Part model, mm, in its own coordinate system. A direction names the side the tool comes from. Give positions to 0.01 mm unless a question says otherwise; leave off trailing zeros. Order: outer loops, then holes, each group sorted by start corner. A loop starts at its lowest first (then second) coordinate and runs counter-clockwise, first axis right, second up.
1. Drop flat-ended pins along their axis: pin 1 Ø1.6 at (x, z) = (-1.5, 1.5) entering from +Y; pin 2 Ø1 at (y, z) = (-10.5, -5.5) entering from +X; pin 3 Ø5 at (x, y) = (-4, -0.25) entering from -Z; pin 4 Ø6 at (x, y) = (-23.5, 5) entering from -Z. Give the stop position or say it passes through.
2. Slice it at A-A on z = -11. List the corners of the cut face in (x, y).
3. Which spindle directions (+Z, -Z, +X, -X, +Y, -Y) get a long thin tool onto all of the face, cutting with end or side? Do faces 1 (the cylindrical face through (-21.797, -0.127, 3.021)), 2 (the cylindrical face through (-20.4, -14.25, -4.3)), 3 (the flat face through (11, 0.75, -6)), 4 (the cylindrical face through (-1.28, 10.24, 0.15)), 5 (the flat face through (-12, 7, -2.25)). Say none if no direction does.
4. Mould opens along Z. For faces 6 (the flat face through (-21, 3.75, 1)), 7 (the flat face through (-12, 5, -2.25)), 8 (the flat face through (-17.8, -1.5, 1.5)), 9 (the flat face through (10, 6.05, -8)) say: +Z half, -Z half, draft (parallel to the pull), parting line (faces both ways), or undercut.
5. Slice it at B-B on y = -20.25. List the corners of the cut face in (x, z), and give its area (3 significant figures).
6. Probe line 1 (Y direction, x = -19, z = 2.35); line 2 (X direction, y = 1, z = 0.25); line 3 (Z direction, x = -10.5, y = -10). List the from-to ranges inside material, lowest first.
7. Slice it at C-C on y = 11. List the corners of the cut face in (x, z) (3 decimals).
from build123d import *

# Parameters (mm, degrees)
BOSS_EXTRUDE1_DEPTH      = 4.5
SKETCH4_W                = 35.509158229
SKETCH4_H                = 48.512063823
CUT_EXTRUDE2_DEPTH       = 10
SKETCH8_W                = 66
SKETCH8_H                = 9
BOSS_EXTRUDE3_DEPTH      = 5
FILLET7_R                = 10
SKETCH16_R               = 1.5
CUT_EXTRUDE6_DEPTH       = 10
SKETCH17_W               = 15.65
SKETCH17_H               = 52.5
CUT_EXTRUDE7_DEPTH       = 10
SKETCH18_R               = 6
CUT_EXTRUDE8_DEPTH       = 10
SKETCH20_W               = 8
SKETCH20_H               = 28
BOSS_EXTRUDE5_DEPTH      = 18
CUT_EXTRUDE10_DEPTH      = 51.084778127
CUT_EXTRUDE10_DEPTH_BACK = 9
SKETCH23_R               = 8
CUT_EXTRUDE11_DEPTH      = 3
CUT_EXTRUDE12_DEPTH      = 68.0001
CUT_EXTRUDE12_DEPTH_BACK = 8
CUT_EXTRUDE12_START      = -42.7
SKETCH24_W               = 11.249996001
SKETCH24_H               = 2
SKETCH25_R               = 1
CUT_EXTRUDE13_DEPTH      = 12.5
CUT_EXTRUDE15_DEPTH      = 2.25
FILLET8_R                = 4
SKETCH27_W               = 21.7
SKETCH27_H               = 7.5
CUT_EXTRUDE16_DEPTH      = 0.4
CHAMFER1_SIZE            = 0.4
CHAMFER2_SIZE            = 0.4
SKETCH28_R               = 2.8
CUT_EXTRUDE17_DEPTH      = 3
SKETCH29_R               = 2
SKETCH29_W               = 21.7
SKETCH29_H               = 0.8
CUT_EXTRUDE18_DEPTH      = 0.4


# Some blends are built 0.0001 mm under size
with BuildPart() as part:
    # Sketch1 → Boss-Extrude1 (new, symmetric)
    with BuildSketch(Plane.XY):
        Polygon((44.5, -23.75), (-0.5, -23.75), (-44.5, -23.75), (-44.5, 23.75), (44.5, 23.75), align=None)
    extrude(amount=BOSS_EXTRUDE1_DEPTH, both=True)

    # Sketch4 → Cut-Extrude2 (cut)
    with BuildSketch(Plane.XY.offset(4.5)):
        with Locations((39.254579115, -0.506031912)):
            Rectangle(SKETCH4_W, SKETCH4_H)
    extrude(amount=-CUT_EXTRUDE2_DEPTH, mode=Mode.SUBTRACT)

    # Sketch8 → Boss-Extrude3 (add)
    with BuildSketch(Plane(origin=(0, 23.75, 0), x_dir=(1, 0, 0), z_dir=(0, 1, 0))):
        with Locations((-11.5, 0)):
            Rectangle(SKETCH8_W, SKETCH8_H)
    extrude(amount=BOSS_EXTRUDE3_DEPTH)

    # Fillet7
    fillet7_edges = [part.edges().sort_by_distance(p)[0] for p in [
        (-44.5, 28.75, 0),
        (21.5, 28.75, 0),
    ]]
    fillet(fillet7_edges, radius=FILLET7_R)

    # Sketch16 → Cut-Extrude6 (cut)
    with BuildSketch(Plane.XY.offset(4.5)):
        with Locations((-19, -0.25)):
            Circle(SKETCH16_R)
        with Locations((-4, -0.25)):
            Circle(SKETCH16_R)
        with Locations((-19, -20.25)):
            Circle(SKETCH16_R)
        with Locations((-4, -20.25)):
            Circle(SKETCH16_R)
    extrude(amount=-CUT_EXTRUDE6_DEPTH, mode=Mode.SUBTRACT)

    # Sketch17 → Cut-Extrude7 (cut)
    with BuildSketch(Plane(origin=(0, 0, -4.5), x_dir=(-1, 0, 0), z_dir=(0, 0, -1))):
        with Locations((36.675, 2.5)):
            Rectangle(SKETCH17_W, SKETCH17_H)
        with Locations((-13.675, 2.5)):
            Rectangle(SKETCH17_W, SKETCH17_H)
    extrude(amount=-CUT_EXTRUDE7_DEPTH, mode=Mode.SUBTRACT)

    # Sketch18 → Cut-Extrude8 (cut)
    with BuildSketch(Plane.XY.offset(4.5)):
        with Locations((-11.5, 16.25)):
            Circle(SKETCH18_R)
    extrude(amount=-CUT_EXTRUDE8_DEPTH, mode=Mode.SUBTRACT)

    # Sketch20 → Boss-Extrude5 (add)
    with BuildSketch(Plane.XY.offset(4.5)):
        with Locations((-32.85, 14.75)):
            Rectangle(SKETCH20_W, SKETCH20_H)
        with Locations((9.85, 14.75)):
            Rectangle(SKETCH20_W, SKETCH20_H)
    extrude(amount=-BOSS_EXTRUDE5_DEPTH)

    # Sketch22 → Cut-Extrude10 (cut, two sides: drawn at the far end of the back side and taken through both)
    with BuildSketch(Plane.XY.offset(4.5).offset(-CUT_EXTRUDE10_DEPTH_BACK)):
        Polygon((-25, 169.372700937), (-25, 28.75), (-25, 16.25), (2, 16.25), (2, 28.75), (2, 169.372700937), (2, 450.61810281), (-25, 450.61810281), align=None)
    extrude(amount=CUT_EXTRUDE10_DEPTH + CUT_EXTRUDE10_DEPTH_BACK, mode=Mode.SUBTRACT)

    # Sketch23 → Cut-Extrude11 (cut)
    with BuildSketch(Plane(origin=(0, 0, -4.5), x_dir=(-1, 0, 0), z_dir=(0, 0, -1))):
        with Locations((11.5, 16.25)):
            Circle(SKETCH23_R)
    extrude(amount=-CUT_EXTRUDE11_DEPTH, mode=Mode.SUBTRACT)

    # Sketch24 → Cut-Extrude12 (cut, two sides: drawn at the far end of the back side and taken through both)
    with BuildSketch(Plane(origin=(13.85, 0, 0), x_dir=(0, 0, -1), z_dir=(1, 0, 0)).offset(CUT_EXTRUDE12_START - CUT_EXTRUDE12_DEPTH_BACK)):
        with Locations((7.875002, 5.05)):
            Rectangle(SKETCH24_W, SKETCH24_H)
    extrude(amount=CUT_EXTRUDE12_DEPTH + CUT_EXTRUDE12_DEPTH_BACK, mode=Mode.SUBTRACT)

    # Sketch25 → Cut-Extrude13 (cut)
    with BuildSketch(Plane(origin=(0, 16.25, 0), x_dir=(1, 0, 0), z_dir=(0, 1, 0))):
        with Locations(Location((-1.5, -1.125, 0), (0, 0, 180))):
            Circle(SKETCH25_R)
        with Locations(Location((-21.5, -1.125, 0), (0, 0, 180))):
            Circle(SKETCH25_R)
    extrude(amount=-CUT_EXTRUDE13_DEPTH, mode=Mode.SUBTRACT)

    # Sketch26 → Cut-Extrude15 (cut)
    with BuildSketch(Plane(origin=(0, 0, -4.5), x_dir=(-1, 0, 0), z_dir=(0, 0, -1))):
        with BuildLine():
            Line((-5.85, 6.05), (28.85, 6.05))
            Line((28.85, 6.05), (28.85, 28.75))
            Line((28.85, 28.75), (25, 28.75))
            Line((25, 28.75), (25, 16.25))
            Line((25, 16.25), (19.5, 16.25))
            ThreePointArc((19.5, 16.25), (11.5, 8.25), (3.5, 16.25))
            Line((3.5, 16.25), (-2, 16.25))
            Line((-2, 16.25), (-2, 28.75))
            Line((-2, 28.75), (-5.85, 28.75))
            Line((-5.85, 28.75), (-5.85, 6.05))
        make_face()
    extrude(amount=-CUT_EXTRUDE15_DEPTH, mode=Mode.SUBTRACT)

    # Fillet8
    # the kernel refuses this fillet: 4 mm, written as the material it adds along each edge
    with BuildSketch(Plane(origin=(-28.85, 0.75, 4.5), x_dir=(-1, 0, 0), z_dir=(0, 0, -1))) as fillet8_piece_1:
        with BuildLine():
            CenterArc((FILLET8_R, -FILLET8_R), FILLET8_R, 90, 90)
            Line((0, -FILLET8_R), (0, 0))
            Line((0, 0), (FILLET8_R, 0))
        make_face()
    extrude(amount=9)
    with BuildSketch(Plane(origin=(5.85, 0.75, 4.5), x_dir=(1, 0, 0), z_dir=(0, 0, -1))) as fillet8_piece_2:
        with BuildLine():
            CenterArc((FILLET8_R, FILLET8_R), FILLET8_R, 180, 90)
            Line((0, FILLET8_R), (0, 0))
            Line((0, 0), (FILLET8_R, 0))
        make_face()
    extrude(amount=9)
    with BuildSketch(Plane(origin=(2, 16.25, -2.25), x_dir=(-1, 0, 0), z_dir=(0, 0, 1))) as fillet8_piece_3_section:
        with BuildLine():
            CenterArc((FILLET8_R, -FILLET8_R), FILLET8_R, 90, 90)
            Line((0, -FILLET8_R), (0, 0))
            Line((0, 0), (FILLET8_R, 0))
        make_face()
    fillet8_piece_3 = extrude(amount=6.75, mode=Mode.PRIVATE)
    fillet8_piece_3 = fillet8_piece_3 - Plane(origin=(-1.5, 17.15044089, 1.125), x_dir=(-1, 0, 0), z_dir=(0, 1, 0)) * Cylinder(1, 30, mode=Mode.PRIVATE)
    add(fillet8_piece_3)
    with BuildSketch(Plane(origin=(-25, 16.25, -2.25), x_dir=(0, 1, 0), z_dir=(0, 0, 1))) as fillet8_piece_4_section:
        with BuildLine():
            CenterArc((FILLET8_R, -FILLET8_R), FILLET8_R, 90, 90)
            Line((0, -FILLET8_R), (0, 0))
            Line((0, 0), (FILLET8_R, 0))
        make_face()
    fillet8_piece_4 = extrude(amount=6.75, mode=Mode.PRIVATE)
    fillet8_piece_4 = fillet8_piece_4 - Plane(origin=(-21.5, 17.150440868, 1.125), x_dir=(-1, 0, 0), z_dir=(0, 1, 0)) * Cylinder(1, 30, mode=Mode.PRIVATE)
    add(fillet8_piece_4)

    # Sketch27 → Cut-Extrude16 (cut)
    with BuildSketch(Plane(origin=(0, 0, -4.5), x_dir=(-1, 0, 0), z_dir=(0, 0, -1))):
        with Locations((11.5, -20)):
            Rectangle(SKETCH27_W, SKETCH27_H)
        with Locations((11.5, -0.5)):
            Rectangle(SKETCH27_W, SKETCH27_H)
    extrude(amount=-CUT_EXTRUDE16_DEPTH, mode=Mode.SUBTRACT)

    # Chamfer1
    chamfer1_edges = [part.edges().sort_by_distance(p)[0] for p in [
        (-11.5, -4.25, -4.1),
    ]]
    chamfer(chamfer1_edges, length=CHAMFER1_SIZE - 0.0001)  # a hair under: the kernel refuses the full size

    # Chamfer2
    chamfer2_edges = [part.edges().sort_by_distance(p)[0] for p in [
        (-11.5, -16.25, -4.1),
    ]]
    chamfer(chamfer2_edges, length=CHAMFER2_SIZE - 0.0001)  # a hair under: the kernel refuses the full size

    # Sketch28 → Cut-Extrude17 (cut)
    with BuildSketch(Plane.XY.offset(4.5)):
        with Locations((-19, -0.25)):
            Circle(SKETCH28_R)
        with Locations((-4, -0.25)):
            Circle(SKETCH28_R)
        with Locations((-4, -20.25)):
            Circle(SKETCH28_R)
        with Locations((-19, -20.25)):
            Circle(SKETCH28_R)
    extrude(amount=-CUT_EXTRUDE17_DEPTH, mode=Mode.SUBTRACT)

    # Sketch29 → Cut-Extrude18 (cut)
    with BuildSketch(Plane(origin=(0, 0, -4.5), x_dir=(-1, 0, 0), z_dir=(0, 0, -1))):
        with Locations((2.65, -4.25)):
            Circle(SKETCH29_R)
        with Locations((20.35, -4.25)):
            Circle(SKETCH29_R)
        with Locations((2.65, -16.25)):
            Circle(SKETCH29_R)
        with Locations((20.35, -16.25)):
            Circle(SKETCH29_R)
        with Locations((11.5, 3.65)):
            Rectangle(SKETCH29_W, SKETCH29_H)
    extrude(amount=-CUT_EXTRUDE18_DEPTH, mode=Mode.SUBTRACT)


solid = part.part
Data:
1. pin 1: stops at y = 16.45
1. pin 2: passes through
1. pin 3: stops at z = -4.1
1. pin 4: stops at z = -4.5
2. outline: (-36.85, 0.75) - (-28.85, 0.75) - (-28.85, 4.05) - (-36.85, 4.05) - close; (-36.85, 6.05) - (-28.85, 6.05) - (-28.85, 28.75) - (-36.85, 28.75) - close; (5.85, 0.75) - (13.85, 0.75) - (13.85, 4.05) - (5.85, 4.05) - close; (5.85, 6.05) - (13.85, 6.05) - (13.85, 28.75) - (5.85, 28.75) - close
3. face 1: +Z
3. face 2: -Z
3. face 3: -Z, +X, -Y
3. face 4: +Y
3. face 5: -Z, +Y
4. face 6: undercut
4. face 7: -Z half
4. face 8: +Z half
4. face 9: draft
5. outline: (-28.85, -4.5) - (-22.35, -4.5) - (-22.35, -4.1) - (-20.5, -4.1) - (-20.5, 1.5) - (-21.8, 1.5) - (-21.8, 4.5) - (-28.85, 4.5) - close; (-17.5, -4.1) - (-5.5, -4.1) - (-5.5, 1.5) - (-6.8, 1.5) - (-6.8, 4.5) - (-16.2, 4.5) - (-16.2, 1.5) - (-17.5, 1.5) - close; (-2.5, -4.1) - (-0.65, -4.1) - (-0.65, -4.5) - (5.85, -4.5) - (5.85, 4.5) - (-1.2, 4.5) - (-1.2, 1.5) - (-2.5, 1.5) - close
5. area: 236 mm2
6. line 1: y = -23.75 to -23.05, -17.45 to -3.05, 2.55 to 16.25
6. line 2: x = -36.85 to -19.83, -18.17 to -4.83, -3.17 to 13.85
6. line 3: z = -4.5 to 4.5
7. outline: (-36.85, -13.5) - (-28.85, -13.5) - (-28.85, -2.25) - (-17.536, -2.25) - (-17.536, -1.5) - (-14.405, -1.5) - (-14.405, 4.5) - (-36.85, 4.5) - close; (-8.595, -1.5) - (-5.464, -1.5) - (-5.464, -2.25) - (5.85, -2.25) - (5.85, -13.5) - (13.85, -13.5) - (13.85, 4.5) - (-8.595, 4.5) - close; hole circle Ø2 at (-21.5, 1.125); hole circle Ø2 at (-1.5, 1.125)
